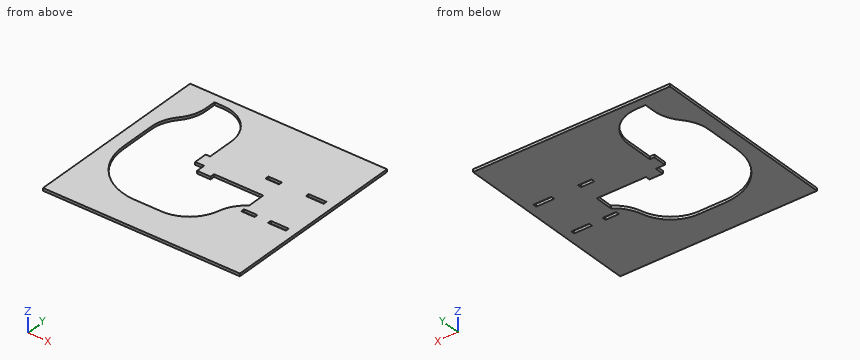
```python
from build123d import *

# Parameters (mm, degrees)
BOSS_EXTRUDE1_DEPTH = 0.15
FILLET3_R           = 6
FILLET4_R           = 4
FILLET5_R           = 4
FILLET7_R           = 4
SKETCH3_W           = 2
SKETCH3_H           = 0.4
SKETCH3_W_2         = 1.5
CUT_EXTRUDE1_DEPTH  = 29.321193478


with BuildPart() as part:
    # Sketch1 → Boss-Extrude1 (new, symmetric)
    with BuildSketch(Plane.XY):
        Polygon((0, 0), (-19, 0), (-19, 21), (0, 21), (3, 21), (3, 0), align=None)
        Polygon((-8.5, 11), (-3, 11), (-3, 9), (-4.5, 9), (-4.5, 3.5), (-17.5, 3.5), (-17.5, 17), (-15.5, 17), (-15.5, 20), (-10.5, 20), (-10.5, 13), (-11, 13), (-11, 11.5), (-10, 11.5), (-10, 10.5), (-8.5, 10.5), align=None, mode=Mode.SUBTRACT)
    extrude(amount=BOSS_EXTRUDE1_DEPTH, both=True)

    # Fillet3
    fillet3_edges = [part.edges().sort_by_distance(p)[0] for p in [
        (-17.5, 3.5, 0),
    ]]
    fillet(fillet3_edges, radius=FILLET3_R)

    # Fillet4
    # the kernel refuses this fillet: 4 mm, written as the material it adds along each edge
    with BuildSketch(Plane(origin=(-17.5, 17, 0.15), x_dir=(0, -1, 0), z_dir=(0, 0, -1))) as fillet4_piece_1:
        with BuildLine():
            CenterArc((3.464101615, -4), FILLET4_R, 90, 60)
            Line((0, -2), (-0.069282032, -1.96))
            ThreePointArc((-0.069282032, -1.96), (-0.08, -1), (-0.08, 0))
            Line((-0.08, 0), (0, 0.08))
            Line((0, 0.08), (3.464101615, 0.08))
            Line((3.464101615, 0.08), (3.464101615, 0))
        make_face()
    extrude(amount=0.3)
    with BuildSketch(Plane(origin=(-4.5, 3.5, 0.15), x_dir=(-1, 0, 0), z_dir=(0, 0, -1))) as fillet4_piece_2:
        with BuildLine():
            CenterArc((FILLET4_R, FILLET4_R), FILLET4_R, 180, 90)
            Line((0, FILLET4_R), (-FILLET4_R * 0.02, FILLET4_R))
            Line((-FILLET4_R * 0.02, FILLET4_R), (-FILLET4_R * 0.02, -FILLET4_R * 0.02))
            Line((-FILLET4_R * 0.02, -FILLET4_R * 0.02), (FILLET4_R, -FILLET4_R * 0.02))
            Line((FILLET4_R, -FILLET4_R * 0.02), (FILLET4_R, 0))
        make_face()
    extrude(amount=0.3)

    # Fillet5
    # the kernel refuses this fillet: 4 mm, written as the material it takes off along each edge
    with BuildSketch(Plane(origin=(-15.5, 17, 4.718502517), x_dir=(0, 1, 0), z_dir=(0, 0, -1))) as fillet5_piece_1:
        with BuildLine():
            CenterArc((1.827401007, -4), FILLET5_R, 90, 41.409622109)
            Line((-0.818350304, -1), (-0.87126533, -0.94))
            ThreePointArc((-0.87126533, -0.94), (-0.430439522, -0.482598297), (-0.069282032, 0.04))
            Line((-0.069282032, 0.04), (0, 0.08))
            Line((0, 0.08), (1.827401007, 0.08))
            Line((1.827401007, 0.08), (1.827401007, 0))
        make_face()
    extrude(amount=9.437005035, mode=Mode.SUBTRACT)
    with BuildSketch(Plane(origin=(-4.5, 9, 6.119736906), x_dir=(-0.041592927859064134, -0.9991346397518759, 0), z_dir=(0, 0, -1))) as fillet5_piece_2:
        with BuildLine():
            CenterArc((3.110715854, -3.934149167), FILLET5_R, 100.410842639, 42.081908104)
            Line((-0.062389392, -1.49870196), (-0.379699916, -1.255157239))
            ThreePointArc((-0.379699916, -1.255157239), (-0.430848552, -0.732713809), (-0.399653856, 0.016637171))
            Line((-0.399653856, 0.016637171), (0.016637171, 0.399653856))
            ThreePointArc((0.016637171, 0.399653856), (1.515339131, 0.337264464), (2.315612653, 0.393414917))
            Line((2.315612653, 0.393414917), (2.387894762, 0))
        make_face()
    extrude(amount=12.239473812, mode=Mode.SUBTRACT)

    # Fillet7
    fillet7_edges = [part.edges().sort_by_distance(p)[0] for p in [
        (-10.5, 20, 0),
    ]]
    fillet(fillet7_edges, radius=FILLET7_R)

    # Sketch3 → Cut-Extrude1 (cut, through all)
    with BuildSketch(Plane.XY.offset(0.15)):
        with Locations((1, 8.05)):
            Rectangle(SKETCH3_W, SKETCH3_H)
        with Locations((-2.25, 8.05)):
            Rectangle(SKETCH3_W_2, SKETCH3_H)
        with Locations((1, 13.45)):
            Rectangle(SKETCH3_W, SKETCH3_H)
        with Locations((-3.75, 13.45)):
            Rectangle(SKETCH3_W_2, SKETCH3_H)
    extrude(amount=-CUT_EXTRUDE1_DEPTH, mode=Mode.SUBTRACT)


solid = part.part
```
Here's how the part is built. I have some questions about the finished solid (model axes, mm). Give positions to 0.01 mm unless a question says otherwise; leave off trailing zeros. Order: outer loops, then holes, each group sorted by start corner. A loop starts at its lowest first (then second) coordinate and runs counter-clockwise, first axis right, second up. Notation, with made-up numbers: (78, 53) -> (131, 53) arc R27 cw to (131, 74) -> close; hole circle Ø2 at (67, 88.25). An arc over 180 degrees is marked (long way). Use CSV: the item, a comma, the result in double quotes. Start each with the question number.
Item 1: Suppose I cut it at D-D (z = 0.1). Give the number of separate pieces and of enclosed holes in the cut face, and give its area (3 significant figures).
Item 2: If I drill on probe 1 along Y at (x, z) = (1.5, 0.05); probe 2 along X at (y, z) = (9.75, -0.05); probe 3 along X at (y, z) = (11.25, 0), over which ranges is the centre line in solid material (lowest first)? Write a range as [from, to].
Item 3: Suppose I cut it at A-A (x = -9.75). List the corners of the cut face in (y, z) for me.
Item 4: Suppose I cut it at B-B (y = 12.5). List the corners of the cut face in (x, z) for me, and give its area (3 significant figures).
Item 5: Suppose I cut it at C-C (x = 0.5). List the corners of the cut face in (y, z) for me.
Answer block:
1,separate pieces,"1"
1,enclosed holes,"5"
1,area,"318 mm^2"
2,probe 1,"y = [0, 7.85], [8.25, 13.25], [13.65, 21]"
2,probe 2,"x = [-19, -17.5], [-3, 3]"
2,probe 3,"x = [-19, -17.5], [-10, 3]"
3,outline,"(0, -0.15) -> (3.5, -0.15) -> (3.5, 0.15) -> (0, 0.15) -> close; (10.5, -0.15) -> (21, -0.15) -> (21, 0.15) -> (10.5, 0.15) -> close"
4,outline,"(-19, -0.15) -> (-17.5, -0.15) -> (-17.5, 0.15) -> (-19, 0.15) -> close; (-11, -0.15) -> (3, -0.15) -> (3, 0.15) -> (-11, 0.15) -> close"
4,area,"4.65 mm^2"
5,outline,"(0, -0.15) -> (7.85, -0.15) -> (7.85, 0.15) -> (0, 0.15) -> close; (8.25, -0.15) -> (13.25, -0.15) -> (13.25, 0.15) -> (8.25, 0.15) -> close; (13.65, -0.15) -> (21, -0.15) -> (21, 0.15) -> (13.65, 0.15) -> close"
